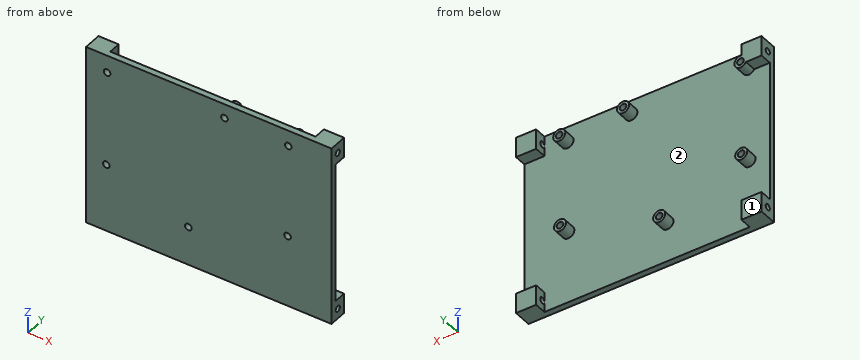
```python
from build123d import *

# Parameters (mm, degrees)
SKETCH1_W           = 122
SKETCH1_H           = 90
BOSS_EXTRUDE1_DEPTH = 3
SKETCH2_R           = 3
SKETCH2_W           = 10
SKETCH2_H           = 10
BOSS_EXTRUDE2_DEPTH = 6
SKETCH3_R           = 1.65
CUT_EXTRUDE1_DEPTH  = 26
CUT_EXTRUDE2_REACH  = 124
SKETCH4_R           = 1.5
CUT_EXTRUDE3_REACH  = 124
SKETCH5_R           = 1.5


with BuildPart() as part:
    # Sketch1 → Boss-Extrude1 (new body)
    with BuildSketch(Plane(origin=(0, 0, 0), x_dir=(1, 0, 0), z_dir=(0, 1, 0))):
        with Locations((61, 45)):
            Rectangle(SKETCH1_W, SKETCH1_H)
    extrude(amount=BOSS_EXTRUDE1_DEPTH)

    # Sketch2 → Boss-Extrude2 (add)
    with BuildSketch(Plane(origin=(0, 3, 0), x_dir=(1, 0, 0), z_dir=(0, 1, 0))):
        with Locations((68.8138, 7.1202)):
            Circle(SKETCH2_R)
        with Locations((100.513, 7.8822)):
            Circle(SKETCH2_R)
        with Locations((10.089, 56.0656)):
            Circle(SKETCH2_R)
        with Locations((100.132, 54.2622)):
            Circle(SKETCH2_R)
        with Locations((50.856, 70.696)):
            Circle(SKETCH2_R)
        with BuildLine():
            Line((0, 0), (10, 0))
            Line((10, 0), (10, 5.706645394))
            ThreePointArc((10, 5.706645394), (13.135115844, 10.046973419), (7.781127404, 10))
            Line((7.781127404, 10), (0, 10))
            Line((0, 10), (0, 0))
        make_face()
        with Locations((5, 85)):
            Rectangle(SKETCH2_W, SKETCH2_H)
        with Locations((117, 85)):
            Rectangle(SKETCH2_W, SKETCH2_H)
        with Locations((117, 5)):
            Rectangle(SKETCH2_W, SKETCH2_H)
    extrude(amount=BOSS_EXTRUDE2_DEPTH)

    # Sketch3 → Cut-Extrude1 (cut)
    with BuildSketch(Plane(origin=(0, 9, 0), x_dir=(1, 0, 0), z_dir=(0, 1, 0))):
        with Locations((10.089, 56.0656)):
            Circle(SKETCH3_R)
        with Locations((50.856, 70.696)):
            Circle(SKETCH3_R)
        with Locations((100.132, 54.2622)):
            Circle(SKETCH3_R)
        with Locations((100.513, 7.8822)):
            Circle(SKETCH3_R)
        with Locations((68.8138, 7.1202)):
            Circle(SKETCH3_R)
        with Locations((10.47, 8.6696)):
            Circle(SKETCH3_R)
    extrude(amount=-CUT_EXTRUDE1_DEPTH, mode=Mode.SUBTRACT)

    # Sketch4 → Cut-Extrude2 (cut, up to next)
    with BuildSketch(Plane.ZY, mode=Mode.PRIVATE) as cut_extrude2_sk1:
        with Locations((-85, 4.5)):
            Circle(SKETCH4_R)
    cut_extrude2_tool1 = extrude(cut_extrude2_sk1.sketch, amount=-CUT_EXTRUDE2_REACH, mode=Mode.PRIVATE) & part.part
    add(cut_extrude2_tool1.solids().sort_by_distance((0, 4.5, -85))[0], mode=Mode.SUBTRACT)
    # Sketch4 → Cut-Extrude2 (cut, up to next)
    with BuildSketch(Plane.ZY, mode=Mode.PRIVATE) as cut_extrude2_sk2:
        with Locations((-5, 4.5)):
            Circle(SKETCH4_R)
    cut_extrude2_tool2 = extrude(cut_extrude2_sk2.sketch, amount=-CUT_EXTRUDE2_REACH, mode=Mode.PRIVATE) & part.part
    add(cut_extrude2_tool2.solids().sort_by_distance((0, 4.5, -5))[0], mode=Mode.SUBTRACT)

    # Sketch5 → Cut-Extrude3 (cut, up to next)
    with BuildSketch(Plane(origin=(122, 0, 0), x_dir=(0, 0, -1), z_dir=(1, 0, 0)), mode=Mode.PRIVATE) as cut_extrude3_sk1:
        with Locations((85, 4.5)):
            Circle(SKETCH5_R)
    cut_extrude3_tool1 = extrude(cut_extrude3_sk1.sketch, amount=-CUT_EXTRUDE3_REACH, mode=Mode.PRIVATE) & part.part
    add(cut_extrude3_tool1.solids().sort_by_distance((122, 4.5, -85))[0], mode=Mode.SUBTRACT)
    # Sketch5 → Cut-Extrude3 (cut, up to next)
    with BuildSketch(Plane(origin=(122, 0, 0), x_dir=(0, 0, -1), z_dir=(1, 0, 0)), mode=Mode.PRIVATE) as cut_extrude3_sk2:
        with Locations((5, 4.5)):
            Circle(SKETCH5_R)
    cut_extrude3_tool2 = extrude(cut_extrude3_sk2.sketch, amount=-CUT_EXTRUDE3_REACH, mode=Mode.PRIVATE) & part.part
    add(cut_extrude3_tool2.solids().sort_by_distance((122, 4.5, -5))[0], mode=Mode.SUBTRACT)


solid = part.part
```
Work out the finished part from the listing and answer in its coordinate system (mm). Face numbers are marked on the shaded views. Give positions to 0.01 mm unless a question says otherwise; leave off trailing zeros. Order: outer loops, then holes, each group sorted by start corner. A loop starts at its lowest first (then second) coordinate and runs counter-clockwise, first axis right, second up. Notation, with made-up numbers: (-35, 73) -> (-7, 73) arc R31 ccw to (-7, 100) -> close; hole circle Ø3 at (-15, 68.25). An arc over 180 degrees is marked (long way). Answer as CSV lines item,"result". Start each with the question number.
(1) Section C-C, the plane x = 26 is taken. Write down the section's boundary in (y, z), plus the area to 3 significant figures.
(2) For a pull along X with two mould halves and no side action, classify the marked faces 1 and 2 as released by +X, released by -X, zero draft, split by the parting line, or undercut.
(3) Section B-B, the plane z = -46.5 is taken. Write down the section's boundary in (x, y).
(4) Consider line 1 along Z through (x, y) = (117.5, 4.5); line 2 along Z through (x, y) = (115, 3.75); line 3 along Y through (x, z) = (7, -5). Determine where each line is inside the solid, lowest interval first.
(5) Each of these flat-tipped pins is pushed along its axis until it touches: pin 1 Ø4 at (x, z) = (56, -49) entering from +Y; pin 2 Ø2 at (x, z) = (100.13, -54.26) entering from -Y; pin 3 Ø1.8 at (y, z) = (4.5, -5) entering from -X; pin 4 Ø1.5 at (x, y) = (101.5, 4.5) entering from -Z. Where does it stop, or does it pass through?
(6) Section A-A, the plane y = 7.5 is taken. Give the number of separate pieces and of enclosed holes in the cut face, plus the area to 3 significant figures.
Entries:
1,outline,"(0, -90) -> (3, -90) -> (3, 0) -> (0, 0) -> close"
1,area,"270 mm²"
2,face 1,"zero draft"
2,face 2,"undercut"
3,outline,"(0, 0) -> (122, 0) -> (122, 3) -> (0, 3) -> close"
4,line 1,"-90 to -86.5, -83.5 to -80, -10 to -6.5, -3.5 to 0"
4,line 2,"-90 to -86.3, -83.7 to -80, -10 to -6.3, -3.7 to 0"
4,line 3,"0 to 3, 6 to 9"
5,pin 1,"y = 3"
5,pin 2,"through"
5,pin 3,"x = 66.07"
5,pin 4,"z = -57.2"
6,separate pieces,"9"
6,enclosed holes,"6"
6,area,"509 mm²"
